Source: CAD feature listing. Evaluate the final solid. Frame: model axes, mm. A direction names the side the tool comes from. Give positions to 0.01 mm unless a question says otherwise; leave off trailing zeros. Loops run counter-clockwise (first coordinate to the right, second up) from the corner with the lowest first, then second, coordinate; pieces in that order, holes last. Notation, with made-up numbers: M 18,74.25 L 41,74.25 A15 ccw 41,92.25 Z; hole C 37.5,44.25 d2. An arc over 180 degrees is marked long. Answer in a Markdown table with one row per item.
```python
from build123d import *

# Parameters (mm, degrees)
BOSS_EXTRUDE2_DEPTH    = 13.80744
CUT_EXTRUDE1_START     = -0.02543021
CUT_EXTRUDE1_OUTLINE_W = 66
CUT_EXTRUDE1_OUTLINE_H = 16
CUT_EXTRUDE1_DEPTH     = 1.106877933
CUT_EXTRUDE2_REACH     = 39.046
SKETCH4_R              = 2.2225


# Read off the part's stored shape, not the designer's step: Cut-Extrude1
with BuildPart() as part:
    # Sketch2 → Boss-Extrude2 (new body)
    with BuildSketch(Plane.XY):
        with BuildLine():
            ThreePointArc((-11.445222977, 4.788221067), (-12.237590886, 2.302953542), (-12.505480711, -0.291778933))
            Line((-12.505480711, -0.291778933), (-7.805480711, -0.291778933))
            ThreePointArc((-7.805480711, -0.291778933), (0.194519289, 7.708221067), (8.194519289, -0.291778933))
            Line((8.194519289, -0.291778933), (12.894519289, -0.291778933))
            ThreePointArc((12.894519289, -0.291778933), (12.626629463, 2.302953542), (11.834261554, 4.788221067))
            ThreePointArc((11.834261554, 4.788221067), (0.194519289, 12.408221067), (-11.445222977, 4.788221067))
        make_face()
        with BuildLine():
            Line((-31.555480711, -0.291778933), (-12.505480711, -0.291778933))
            ThreePointArc((-12.505480711, -0.291778933), (-12.237590886, 2.302953542), (-11.445222977, 4.788221067))
            Line((-11.445222977, 4.788221067), (-31.555480711, 4.788221067))
            Line((-31.555480711, 4.788221067), (-31.555480711, -0.291778933))
        make_face()
        with BuildLine():
            ThreePointArc((11.834261554, 4.788221067), (12.626629463, 2.302953542), (12.894519289, -0.291778933))
            Line((12.894519289, -0.291778933), (31.944519289, -0.291778933))
            Line((31.944519289, -0.291778933), (31.944519289, 4.788221067))
            Line((31.944519289, 4.788221067), (11.834261554, 4.788221067))
        make_face()
    extrude(amount=BOSS_EXTRUDE2_DEPTH)

    # Cut-Extrude1 outline → Cut-Extrude1 (cut)
    with BuildSketch(Plane(origin=(0, 0, 0), x_dir=(1, 0, 0), z_dir=(0, 0.08715574274765836, -0.9961946980917455)).offset(CUT_EXTRUDE1_START)):
        with Locations((0, -6)):
            Rectangle(CUT_EXTRUDE1_OUTLINE_W, CUT_EXTRUDE1_OUTLINE_H)
    extrude(amount=CUT_EXTRUDE1_DEPTH, mode=Mode.SUBTRACT)

    # Sketch4 → Cut-Extrude2 (cut, up to next)
    with BuildSketch(Plane.XZ.offset(0.291778933), mode=Mode.PRIVATE) as cut_extrude2_sk1:
        with Locations(Location((-16.315480711, 7.45744, 0), (0, 0, 270))):
            Circle(SKETCH4_R)
    cut_extrude2_tool1 = extrude(cut_extrude2_sk1.sketch, amount=-CUT_EXTRUDE2_REACH, mode=Mode.PRIVATE) & part.part
    # Sketch4 → Cut-Extrude2 (cut, up to next)
    with BuildSketch(Plane.XZ.offset(0.291778933), mode=Mode.PRIVATE) as cut_extrude2_sk2:
        with Locations(Location((16.704519289, 7.45744, 0), (0, 0, 270))):
            Circle(SKETCH4_R)
    cut_extrude2_tool2 = extrude(cut_extrude2_sk2.sketch, amount=-CUT_EXTRUDE2_REACH, mode=Mode.PRIVATE) & part.part
    add(cut_extrude2_tool1.solids().sort_by_distance((-16.315481, -0.291779, 7.45744))[0], mode=Mode.SUBTRACT)
    add(cut_extrude2_tool2.solids().sort_by_distance((16.704519, -0.291779, 7.45744))[0], mode=Mode.SUBTRACT)


solid = part.part
```
1) Pin query (flat end, axial travel): pin 1 Ø4 at (x, z) = (-20.5, 7) entering from +Y; pin 2 Ø1 at (y, z) = (6, 11) entering from +X; pin 3 Ø6 at (x, z) = (-16.32, 7.46) entering from -Y. Return the tip coordinate at first contact, or that it passes through.
Reply:
| item | result |
|---|---|
| pin 1 | stops at y = 4.79 |
| pin 2 | stops at x = 11.5 |
| pin 3 | stops at y = -0.29 |
2) Section C-C, the plane z = 7.75. Return loops of the section in (x, y), then the cut area to 3 significant figures.
Reply:
| item | result |
|---|---|
| outline | M -31.56,-0.29 L -18.52,-0.29 L -18.52,4.79 L -31.56,4.79 Z; M -14.11,-0.29 L -7.81,-0.29 A8 cw 8.19,-0.29 L 14.5,-0.29 L 14.5,4.79 L 11.83,4.79 A12.7 ccw -11.45,4.79 L -14.11,4.79 Z; M 18.91,-0.29 L 31.94,-0.29 L 31.94,4.79 L 18.91,4.79 Z |
| area | 305 mm² |
3) Pull-direction query (X, two-part tool) for faces 4 (the cylindrical face through (-15.648, 2.213, 5.338)), 5 (the cylindrical face through (0.401, 12.407, 7.032)), 6 (the flat face through (-0.25, 8.792, 0.795)); classes: released by +X, released by -X, zero draft, split by the parting line, or undercut.
Reply:
| item | result |
|---|---|
| face 4 | undercut |
| face 5 | split by the parting line |
| face 6 | zero draft |
4) Set-up query: faces 1 (the flat face through (0, 9, 13.807)), 2 (the flat face through (-21, 4.788, 7)), 3 (the flat face through (22, 4.788, 7)). Return all of +Z, -Z, +X, -X, +Y, -Y with unobstructed straight access to the full face (end or side cutting, diameter ignored); none if empty.
Reply:
| item | result |
|---|---|
| face 1 | +Z, +X, -X, +Y, -Y |
| face 2 | +Z, -Z, -X, +Y |
| face 3 | +Z, -Z, +X, +Y |
5) Section B-B, the plane x = -18. Return loops of the section in (y, z), then the cut area to 3 significant figures.
Reply:
| item | result |
|---|---|
| outline | M -0.29,0 L 4.79,0.44 L 4.79,6.01 L -0.29,6.01 Z; M -0.29,8.91 L 4.79,8.91 L 4.79,13.81 L -0.29,13.81 Z |
| area | 54.3 mm² |
6) Material intervals for L1, parallel to Y at x = 29.5, z = 5; L2, parallel to X at y = 2, z = 3; L3, parallel to Z at x = -17, y = 3.25, sorted ascending.
Reply:
| item | result |
|---|---|
| L1 | y = -0.29 to 4.79 |
| L2 | x = -31.56 to -7.47, 7.86 to 31.94 |
| L3 | z = 0.31 to 5.34, 9.57 to 13.81 |
7) Section A-A, the plane y = 2.5. Return loops of the section in (x, z) (1 decimal), then the cut area to 3 significant figures.
Reply:
| item | result |
|---|---|
| outline | M -31.6,0.2 L -7.3,0.2 L -7.3,13.8 L -31.6,13.8 Z; M 7.7,0.2 L 31.9,0.2 L 31.9,13.8 L 7.7,13.8 Z; hole C -16.3,7.5 d4.4; hole C 16.7,7.5 d4.4 |
| area | 627 mm² |
8) Section D-D, the plane y = 6.5. Return loops of the section in (x, z), then the cut area to 3 significant figures.
Reply:
| item | result |
|---|---|
| outline | M -10.54,0.59 L -4.03,0.59 L -4.03,13.81 L -10.54,13.81 Z; M 4.42,0.59 L 10.93,0.59 L 10.93,13.81 L 4.42,13.81 Z |
| area | 172 mm² |
